Input: part model. Units: mm. Frame: model coordinates. A direction names the side the tool comes from. Coordinates: 2 decimals unless noted, no trailing zeros. Loops run counter-clockwise (first coordinate to the right, second up) from the corner with the lowest first, then second, coordinate; pieces in that order, holes last.
```python
from build123d import *

# Parameters (mm, degrees)
SKETCH1_W           = 50.8
SKETCH1_H           = 61.92
BOSS_EXTRUDE2_DEPTH = 6.35
SKETCH2_R           = 16
CUT_EXTRUDE1_DEPTH  = 7.35
CUT_EXTRUDE4_DEPTH  = 7.35
CUT_EXTRUDE5_REACH  = 8.35
SKETCH5_R           = 2.75
FILLET1_R           = 1


with BuildPart() as part:
    # Sketch1 → Boss-Extrude2 (new body)
    with BuildSketch(Plane(origin=(0, 0, 0), x_dir=(0, 0, -1), z_dir=(1, 0, 0))):
        with Locations((25.4, 30.96)):
            Rectangle(SKETCH1_W, SKETCH1_H)
    extrude(amount=BOSS_EXTRUDE2_DEPTH)

    # Sketch2 → Cut-Extrude1 (cut, through all)
    with BuildSketch(Plane.ZY):
        with Locations((-25.4, 30.960695)):
            Circle(SKETCH2_R)
    extrude(amount=-CUT_EXTRUDE1_DEPTH, mode=Mode.SUBTRACT)

    # Sketch4 → Cut-Extrude4 (cut, through all)
    with BuildSketch(Plane(origin=(6.35, 0, 0), x_dir=(0, 0, -1), z_dir=(1, 0, 0))):
        Polygon((11.4, 59.839253392), (11.4, 37.92), (39.4, 37.92), (39.4, 59.62), (30.034684812, 59.62), (33.389978254, 65.431538715), (18.305977376, 65.431538715), (21.534684812, 59.839253392), align=None)
    extrude(amount=-CUT_EXTRUDE4_DEPTH, mode=Mode.SUBTRACT)

    # Sketch5 → Cut-Extrude5 (cut, up to next)
    with BuildSketch(Plane.ZY, mode=Mode.PRIVATE) as cut_extrude5_sk1:
        with Locations((-45.795509398, 5.272471121)):
            Circle(SKETCH5_R)
    cut_extrude5_tool1 = extrude(cut_extrude5_sk1.sketch, amount=-CUT_EXTRUDE5_REACH, mode=Mode.PRIVATE) & part.part
    add(cut_extrude5_tool1.solids().sort_by_distance((0, 5.272471, -45.795509))[0], mode=Mode.SUBTRACT)
    # Sketch5 → Cut-Extrude5 (cut, up to next)
    with BuildSketch(Plane.ZY, mode=Mode.PRIVATE) as cut_extrude5_sk2:
        with Locations((-25.399655405, 5.560695)):
            Circle(SKETCH5_R)
    cut_extrude5_tool2 = extrude(cut_extrude5_sk2.sketch, amount=-CUT_EXTRUDE5_REACH, mode=Mode.PRIVATE) & part.part
    add(cut_extrude5_tool2.solids().sort_by_distance((0, 5.560695, -25.399655))[0], mode=Mode.SUBTRACT)
    # Sketch5 → Cut-Extrude5 (cut, up to next)
    with BuildSketch(Plane.ZY, mode=Mode.PRIVATE) as cut_extrude5_sk3:
        with Locations((-7.439487758, 13.000182758)):
            Circle(SKETCH5_R)
    cut_extrude5_tool3 = extrude(cut_extrude5_sk3.sketch, amount=-CUT_EXTRUDE5_REACH, mode=Mode.PRIVATE) & part.part
    add(cut_extrude5_tool3.solids().sort_by_distance((0, 13.000183, -7.439488))[0], mode=Mode.SUBTRACT)
    # Sketch5 → Cut-Extrude5 (cut, up to next)
    with BuildSketch(Plane.ZY, mode=Mode.PRIVATE) as cut_extrude5_sk4:
        with Locations((-43.35992398, 48.920755906)):
            Circle(SKETCH5_R)
    cut_extrude5_tool4 = extrude(cut_extrude5_sk4.sketch, amount=-CUT_EXTRUDE5_REACH, mode=Mode.PRIVATE) & part.part
    add(cut_extrude5_tool4.solids().sort_by_distance((0, 48.920756, -43.359924))[0], mode=Mode.SUBTRACT)
    # Sketch5 → Cut-Extrude5 (cut, up to next)
    with BuildSketch(Plane.ZY, mode=Mode.PRIVATE) as cut_extrude5_sk5:
        with Locations((-5.004504526, 56.648087135)):
            Circle(SKETCH5_R)
    cut_extrude5_tool5 = extrude(cut_extrude5_sk5.sketch, amount=-CUT_EXTRUDE5_REACH, mode=Mode.PRIVATE) & part.part
    add(cut_extrude5_tool5.solids().sort_by_distance((0, 56.648087, -5.004505))[0], mode=Mode.SUBTRACT)

    # Fillet1
    fillet1_edges = [part.edges().sort_by_distance(p)[0] for p in [
        (3.175, 59.62, -39.4),
        (3.175, 59.839253392, -11.4),
    ]]
    fillet(fillet1_edges, radius=FILLET1_R)


solid = part.part
```
Item 1: Section query B-B (z = -25.4). Output: boundary loops of the cut face in (x, y), then the cut area to 3 significant figures.
Result:
outline: (0, 0) - (6.35, 0) - (6.35, 2.81) - (0, 2.81) - close; (0, 8.31) - (6.35, 8.31) - (6.35, 14.96) - (0, 14.96) - close
area: 60.1 mm2
Item 2: Section query A-A (y = 43). Output: boundary loops of the cut face in (x, z).
Result:
outline: (0, -50.8) - (6.35, -50.8) - (6.35, -39.4) - (0, -39.4) - close; (0, -11.4) - (6.35, -11.4) - (6.35, 0) - (0, 0) - close
Item 3: Section query C-C (x = 1.5). Output: boundary loops of the cut face in (y, z), then the cut area to 3 significant figures.
Result:
outline: (0, -50.8) - (61.92, -50.8) - (61.92, -31.36) - (59.62, -30.03) - (59.62, -38.4) arc R1 cw to (58.62, -39.4) - (38.71, -39.4) arc R16 cw (long way) to (38.71, -11.4) - (58.84, -11.4) arc R1 cw to (59.84, -12.4) - (59.84, -21.53) - (61.92, -20.33) - (61.92, 0) - (0, 0) - close; hole circle Ø5.5 at (5.27, -45.8); hole circle Ø5.5 at (5.56, -25.4); hole circle Ø5.5 at (13, -7.44); hole circle Ø5.5 at (48.92, -43.36); hole circle Ø5.5 at (56.65, -5)
area: 1,780 mm2
Item 4: Line query: L1, parallel to Z at x = 1, y = 26; L2, parallel to Y at x = 4.75, z = -25.4; L3, parallel to Y at x = 5.25, z = -5.5. Output: solid intervals per line, ascending.
Result:
L1: z = -50.8 to -40.61, -10.19 to 0
L2: y = 0 to 2.81, 8.31 to 14.96
L3: y = 0 to 11.05, 14.95 to 53.94, 59.35 to 61.92
Item 5: Reachability of faces 1 (the face through (3.22, 60.89, -20.93)), 2 (the face through (3, 49, -39.4)), 3 (the face through (0, 18, -14)) from +Z, -Z, +X, -X, +Y, -Y: full face, straight path, thin tool, end or side. Return the list, or none.
Result:
face 1: +X, -X, +Y
face 2: +X, -X
face 3: +Z, -Z, -X, +Y, -Y
Item 6: Contact query for a flat-ended pin moving along its axis: P1, Ø3.5, axis at y = 56.65, z = -5, coming from the -X side (3 decimals). Output: stop coordinate, or through.
Result:
P1: passes through
Item 7: Mould query, pull axis Z, two halves, no side actions, for faces 4 (the face through (3, 59.839, -17)), 5 (the face through (3, 31, -50.8)), 6 (the face through (3.131, 14.967, -25.865)), 7 (the face through (3, 31, 0)). Classes: +Z half, -Z half, draft (parallel to the pull), parting line (faces both ways), or undercut.
Result:
face 4: undercut
face 5: -Z half
face 6: undercut
face 7: +Z half
